Autodesk Inventor part; units mm, degrees
ref_plane "YZ Plane" through (0, 0, 0) normal (1, 0, 0) x (0, 1, 0)
ref_plane "XZ Plane" through (0, 0, 0) normal (0, 1, 0) x (-1, 0, 0)
ref_plane "XY Plane" through (0, 0, 0) normal (0, 0, 1) x (1, 0, 0)
sketch "Sketch1" plane through (0, 0, 0) normal (0, 0, 1) x (1, 0, 0)
  line L0 (-140.3442, -2139.338) -> (951.8558, -2139.338)
  line L1 (951.8558, -2139.338) -> (951.8558, -158.138)
  line L2 (951.8558, -158.138) -> (-140.3442, -158.138)
  line L3 (-140.3442, -158.138) -> (-140.3442, -2139.338)
  line L4 (253.3558, -488.338) -> (558.1558, -488.338)
  line L5 (558.1558, -488.338) -> (558.1558, -564.538)
  line L6 (558.1558, -564.538) -> (253.3558, -564.538)
  line L7 (253.3558, -564.538) -> (253.3558, -488.338)
  line L8 (253.3558, -996.338) -> (558.1558, -996.338)
  line L9 (558.1558, -996.338) -> (558.1558, -1072.538)
  line L10 (558.1558, -1072.538) -> (253.3558, -1072.538)
  line L11 (253.3558, -1072.538) -> (253.3558, -996.338)
  line L12 (253.3558, -1504.338) -> (558.1558, -1504.338)
  line L13 (558.1558, -1504.338) -> (558.1558, -1580.538)
  line L14 (558.1558, -1580.538) -> (253.3558, -1580.538)
  line L15 (253.3558, -1580.538) -> (253.3558, -1504.338)
  point P0 (0, 0)
  dimension "d0" = 1092.2
  dimension "d1" = 1981.2
  dimension "d2" = 393.7
  dimension "d3" = 393.7
  dimension "d4" = 393.7
  dimension "d5" = 304.8
  dimension "d6" = 304.8
  dimension "d7" = 304.8
  dimension "d8" = 76.2
  dimension "d9" = 76.2
  dimension "d10" = 76.2
  dimension "d11" = 558.8
  dimension "d12" = 1066.8
  dimension "d13" = 1574.8
extrude "Extrusion1" add sketch "Sketch1" against normal blind 19.05
sketch "Sketch2" plane through (-140.3442, -2139.338, 0) normal (0, -1, 0) x (1, 0, 0)
  line L0 (0, -19.05) -> (1092.2, -19.05)
  line L1 (1092.2, 0) -> (1092.2, -19.05)
  line L2 (0, 0) -> (1092.2, 0)
  line L3 (0, 0) -> (0, -19.05)
  line L4 (0, -19.05) -> (1092.2, -19.05)
  line L5 (1092.2, 0) -> (1092.2, -19.05)
  line L6 (0, 0) -> (1092.2, 0)
  line L7 (0, 0) -> (0, -19.05)
  line L8 (1092.2, 28.575) -> (0, 28.575)
  line L9 (0, 28.575) -> (0, -47.625)
  line L10 (0, -47.625) -> (1092.2, -47.625)
  line L11 (1092.2, -47.625) -> (1092.2, 28.575)
  point P0 (140.3442, 0)
  dimension "d16" = 76.2
  dimension "d17" = 28.575
extrude "Extrusion2" add sketch "Sketch2" against normal blind 19.05 contours L0 L11 L10 L9 | L9 L8 L11 L2
sketch "Sketch3" plane through (0, 0, -19.05) normal (0, 0, -1) x (-1, 0, 0)
  line L0 (-253.3558, -996.338) -> (-253.3558, -1072.538)
  line L1 (-253.3558, -1072.538) -> (-558.1558, -1072.538)
  line L2 (-558.1558, -1072.538) -> (-558.1558, -996.338)
  line L3 (-253.3558, -488.338) -> (-253.3558, -564.538)
  line L4 (-253.3558, -564.538) -> (-558.1558, -564.538)
  line L5 (-558.1558, -564.538) -> (-558.1558, -488.338)
  line L6 (-253.3558, -1504.338) -> (-253.3558, -1580.538)
  line L7 (-253.3558, -1580.538) -> (-558.1558, -1580.538)
  line L8 (-558.1558, -1580.538) -> (-558.1558, -1504.338)
  point P0 (0, 0)
  point P1 (-507.3558, -589.938)
  point P2 (-304.1558, -589.938)
  point P3 (-507.3558, -1097.938)
  point P4 (-304.1558, -1097.938)
  point P5 (-507.3558, -1605.938)
  point P6 (-304.1558, -1605.938)
  dimension "d20" = 50.8
  dimension "d21" = 50.8
  dimension "d22" = 25.4
  dimension "d23" = 25.4
  dimension "d24" = 50.8
  dimension "d25" = 50.8
  dimension "d26" = 25.4
  dimension "d27" = 25.4
  dimension "d28" = 50.8
  dimension "d29" = 25.4
  dimension "d30" = 50.8
  dimension "d31" = 25.4
hole "Hole1" at (507.3558, -589.938, -19.05) at (304.1558, -589.938, -19.05) at (507.3558, -1097.938, -19.05) at (304.1558, -1097.938, -19.05) at (507.3558, -1605.938, -19.05) at (304.1558, -1605.938, -19.05) direction (0, 0, 1) diameter 6.858 depth 25.4 tip angle 118
thread "Thread1"
thread "Thread2"
thread "Thread3"
thread "Thread4"
thread "Thread5"
thread "Thread6"
equation "\"d6\" = d5"
equation "\"d7\" = d5"
equation "\"d9\" = d8"
equation "\"d10\" = d8"
properties part number "feederStationSlots"
CAD build for the part. Positions are in the model's coordinates, mm. A direction names the side the tool comes from. Coordinates: 2 decimals unless noted, no trailing zeros. Loops run counter-clockwise (first coordinate to the right, second up) from the corner with the lowest first, then second, coordinate; pieces in that order, holes last. Notation, with made-up numbers: (61.5, 42) - (107.5, 42) arc R8 cw to (107.5, 52) - close; hole circle Ø9 at (63, 23.5). An arc over 180 degrees is marked (long way). Return JSON: item names as keys, results as strings.
1. Band-saw the part on D-D (y = -370). Give the cut face in (x, z), and give its area (3 significant figures).
Result:
{"outline": "(-140.34, -19.05) - (951.86, -19.05) - (951.86, 0) - (-140.34, 0) - close", "area": "20,800 mm2"}
2. Probe L1, parallel to Y at x = 377.5, z = -5; L2, parallel to Z at x = 512, y = -1177; L3, parallel to Y at x = 737, z = -25. List the from-to ranges inside material, lowest first. Write a range as from..to.
Result:
{"L1": "y = -2139.34..-1580.54, -1504.34..-1072.54, -996.34..-564.54, -488.34..-158.14", "L2": "z = -19.05..0", "L3": "y = -2139.34..-2120.29"}
3. 3-axis set-ups, long thin cutter, end or side, ignore diameter. For faces 1 (the flat face through (398, -1125, -19.05)), 2 (the flat face through (951.856, -1153, -7)), 3 (the flat face through (398, -1125, 0)): which of +Z, -Z, +X, -X, +Y, -Y reach the whole face in a straight line?
Result:
{"face 1": "-Z, +X, -X, +Y", "face 2": "+Z, -Z, +X, +Y, -Y", "face 3": "+Z, +X, -X, +Y"}
4. Drop flat-ended pins along their axis: pin 1 (5.5 mm diameter, centred on x = 304.16, y = -589.94, fed in from -Z); pin 2 (1 mm diameter, centred on x = 345, y = -900.5, fed in from +Z); pin 3 (4 mm diameter, centred on x = 16, y = -1368.5, fed in from -Z). Give the stop position or say it passes through.
Result:
{"pin 1": "passes through", "pin 2": "stops at z = 0", "pin 3": "stops at z = -19.05"}
5. Band-saw the part on A-A (x = 387.5). Give the cut face in (y, z) (3 decimals).
Result:
{"outline": "(-2139.338, -47.625) - (-2120.288, -47.625) - (-2120.288, -19.05) - (-1580.538, -19.05) - (-1580.538, 0) - (-2120.288, 0) - (-2120.288, 28.575) - (-2139.338, 28.575) - close; (-1504.338, -19.05) - (-1072.538, -19.05) - (-1072.538, 0) - (-1504.338, 0) - close; (-996.338, -19.05) - (-564.538, -19.05) - (-564.538, 0) - (-996.338, 0) - close; (-488.338, -19.05) - (-158.138, -19.05) - (-158.138, 0) - (-488.338, 0) - close"}
6. Band-saw the part on B-B (x = -13.5). Give the cut face in (y, z) (3 decimals), and give its area (3 significant figures).
Result:
{"outline": "(-2139.338, -47.625) - (-2120.288, -47.625) - (-2120.288, -19.05) - (-158.138, -19.05) - (-158.138, 0) - (-2120.288, 0) - (-2120.288, 28.575) - (-2139.338, 28.575) - close", "area": "38,800 mm2"}
7. Band-saw the part on C-C (z = 13.5). Give the cut face in (x, y).
Result:
{"outline": "(-140.34, -2139.34) - (951.86, -2139.34) - (951.86, -2120.29) - (-140.34, -2120.29) - close"}
